Job drawing, mm, ordinate dimensions from the low corner. One solid piece. A direction names the side the tool comes from. Coordinates: 2 decimals unless noted, no trailing zeros. Order: outer loops, then holes, each group sorted by start corner. A loop starts at its lowest first (then second) coordinate and runs counter-clockwise, first axis right, second up. Notation, with made-up numbers: (-38.75, 79) - (11.25, 79) arc R28 ccw to (11.25, 118) - close; hole circle Ø10 at (79, -9.75). An arc over 180 degrees is marked (long way). Use a Markdown table: item, result. Add a question column.
1) Tool access for the marked faces 1 and 2: list every direction of +Z, -Z, +X, -X, +Y, -Y with a clear straight run to the whole face (end or side of a thin tool).
2) Saw through at B-B on x = 37.5. List the corners of the cut face in (y, z).
3) Drop flat-ended pins along their axis: P1, Ø8.5, axis at x = 37.5, z = 11.25, coming from the +Y side; P2, Ø7, axis at y = 19.5, z = 15, coming from the +X side; P3, Ø6, axis at x = 12.5, z = 11.25, coming from the +Y side. Give the stop position or say it passes through.
4) Saw through at D-D on z = 4.75. List the corners of the cut face in (x, y), then the cut area to 3 significant figures.
5) Wall check: L1, parallel to Z at x = 12.5, y = 1.7; L2, parallel to Y at x = 3.6, z = 11.25; L3, parallel to Y at x = 3.1, z = 11.25. Give the ranges that are in metal, low to high. Write a range as [from, to].
6) Saw through at A-A on z = 11.25. List the corners of the cut face in (x, y).
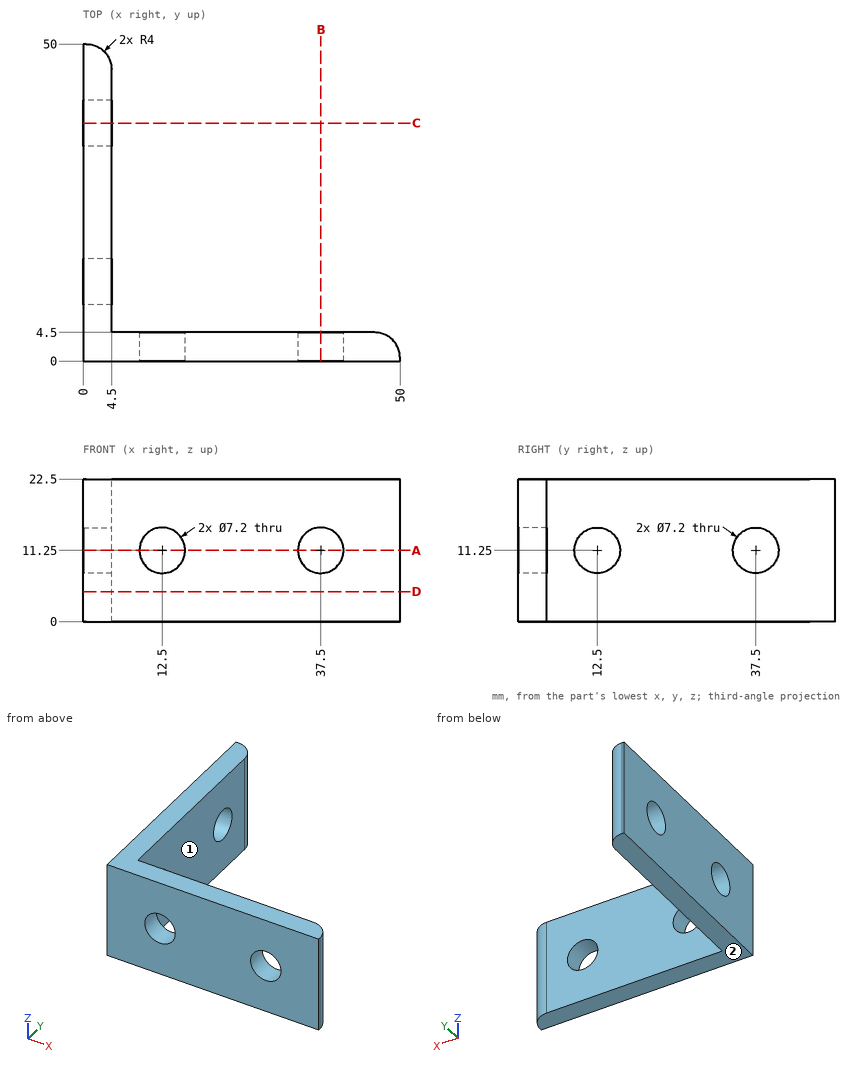
Results are:
| question | item | result |
|---|---|---|
| 1 | face 1 | +Z, -Z, +X, +Y |
| 1 | face 2 | -Z, +X, -X, +Y, -Y |
| 2 | outline | (0, 0) - (4.5, 0) - (4.5, 7.65) - (0, 7.65) - close; (0, 14.85) - (4.5, 14.85) - (4.5, 22.5) - (0, 22.5) - close |
| 3 | P1 | y = 4.5 |
| 3 | P2 | x = 4.5 |
| 3 | P3 | through |
| 4 | outline | (0, 0) - (50, 0) - (50, 0.5) arc R4 ccw to (46, 4.5) - (4.5, 4.5) - (4.5, 46) arc R4 ccw to (0.5, 50) - (0, 50) - close |
| 4 | area | 423 mm2 |
| 5 | L1 | [0, 7.65], [14.85, 22.5] |
| 5 | L2 | [0, 8.9], [16.1, 33.9], [41.1, 48.53] |
| 5 | L3 | [0, 8.9], [16.1, 33.9], [41.1, 49.04] |
| 6 | outline | (0, 0) - (8.9, 0) - (8.9, 4.5) - (4.5, 4.5) - (4.5, 8.9) - (0, 8.9) - close; (0, 16.1) - (4.5, 16.1) - (4.5, 33.9) - (0, 33.9) - close; (0, 41.1) - (4.5, 41.1) - (4.5, 46) arc R4 ccw to (0.5, 50) - (0, 50) - close; (16.1, 0) - (33.9, 0) - (33.9, 4.5) - (16.1, 4.5) - close; (41.1, 0) - (50, 0) - (50, 0.5) arc R4 ccw to (46, 4.5) - (41.1, 4.5) - close |
